Autodesk Inventor part; units mm, degrees
ref_plane "YZ Plane" through (0, 0, 0) normal (1, 0, 0) x (0, 1, 0)
ref_plane "XZ Plane" through (0, 0, 0) normal (0, 1, 0) x (-1, 0, 0)
ref_plane "XY Plane" through (0, 0, 0) normal (0, 0, 1) x (1, 0, 0)
sketch "Sketch1" plane through (0, 0, 0) normal (0, 0, 1) x (1, 0, 0)
  line L0 (0, 0) -> (0, 15)
  line L1 (0, 0) -> (15, 0)
  arc A0 (15, 0) -> (0, 15) centre (0, 0) ccw
  line L2 (0, -3.6213) -> (0, 21.7279)
  dimension "d2" = 15
revolve "Revolution1" add sketch "Sketch1" angle 360 about axis through (0, -10, 0) along (0, 1, 0)
sketch "Sketch4" plane through (0, 0, 0) normal (0, -1, 0) x (1, 0, 0)
  point P0 (0, 0)
  point P1 (0, 0)
hole "Hole2" at (0, 0, 0) direction (0, 1, 0) diameter 3.242 depth 11.8 tip angle 118
shell "Shell2" thickness 3 removed faces 1 at (10.3911, 0, 1.2617)
properties part number "Ball_Upper Half" material "Nylon 6/6"
Geometry check sheet. Reference: the model listing, model coordinates, mm. A direction names the side the tool comes from. Round coordinates to 2 decimals unless told otherwise and drop trailing zeros. Loops run counter-clockwise (first coordinate to the right, second up) from the corner with the lowest first, then second, coordinate; pieces in that order, holes last. Notation, with made-up numbers: (-21, 45) - (28, 45) arc R19 cw to (28, 72) - close; hole circle Ø3 at (-39.75, 67). An arc over 180 degrees is marked (long way). Answer as CSV lines item,"result".
(1) Set-up check for faces 3 (the face through (4.51, 5.61, 1)), 4 (the face through (7, 0, -10)): record each of +Z, -Z, +X, -X, +Y, -Y from which the full face is reachable in a straight line by a thin tool's end or side.
Output values:
face 3,"-Y"
face 4,"+Z, -Z, +X, -X, -Y"
(2) Release check for a two-part mould opening along X. For faces 1 (the face through (0, 0, 2)), 2 (the face through (1.438, 5.983, -0.748)) record: released by +X, released by -X, zero draft, split by the parting line, or undercut.
Output values:
face 1,"zero draft"
face 2,"undercut"
(3) Depth check by flat-ended pin: pin 1 Ø4 at (y, z) = (3, 5) entering from +X; pin 2 Ø2 at (y, z) = (9.5, -5.5) entering from +X; pin 3 Ø3 at (x, z) = (-7.5, 4.5) entering from -Y. Enter the tip coordinate at first touch or a pass-through.
Output values:
pin 1,"stops at x = 14.5"
pin 2,"stops at x = 11.2"
pin 3,"stops at y = 6.25"
(4) Cross-section at B-B, the plane x = 2.5. Enter the section's corners in (y, z), and give its area (3 significant figures).
Output values:
outline,"(0, -14.79) arc R14.79 ccw to (0, 14.79) - (0, 11.74) arc R11.74 cw to (11.07, 3.89) - (0, 3.89) - (0, -3.89) - (11.07, -3.89) arc R11.74 cw to (0, -11.74) - close"
area,"217 mm²"
(5) Cross-section at A-A, the plane y = 1. Enter the section's corners in (x, z).
Output values:
outline,"circle Ø29.93 at (0, 0); circle Ø9.24 at (0, 0); hole circle Ø23.92 at (0, 0); hole circle Ø3.24 at (0, 0)"
(6) Cross-section at D-D, the plane y = 13.5. Enter the section's corners in (x, z).
Output values:
outline,"circle Ø13.08 at (0, 0)"
(7) Cross-section at C-C, the plane z = 11.5. Enter the section's corners in (x, y), and give its area (3 significant figures).
Output values:
outline,"(-9.63, 0) - (-3.43, 0) arc R3.43 cw to (3.43, 0) - (9.63, 0) arc R9.63 ccw to start"
area,"127 mm²"
(8) Material ranges on line 1 along X through (y, z) = (8.5, -0.5); line 2 along Z through (x, y) = (0, 4), recorded low to high.
Output values:
line 1,"x = -12.35 to -8.46, -4.59 to -1.54, 1.54 to 4.59, 8.46 to 12.35"
line 2,"z = -14.46 to -11.31, -4.62 to -1.62, 1.62 to 4.62, 11.31 to 14.46"
